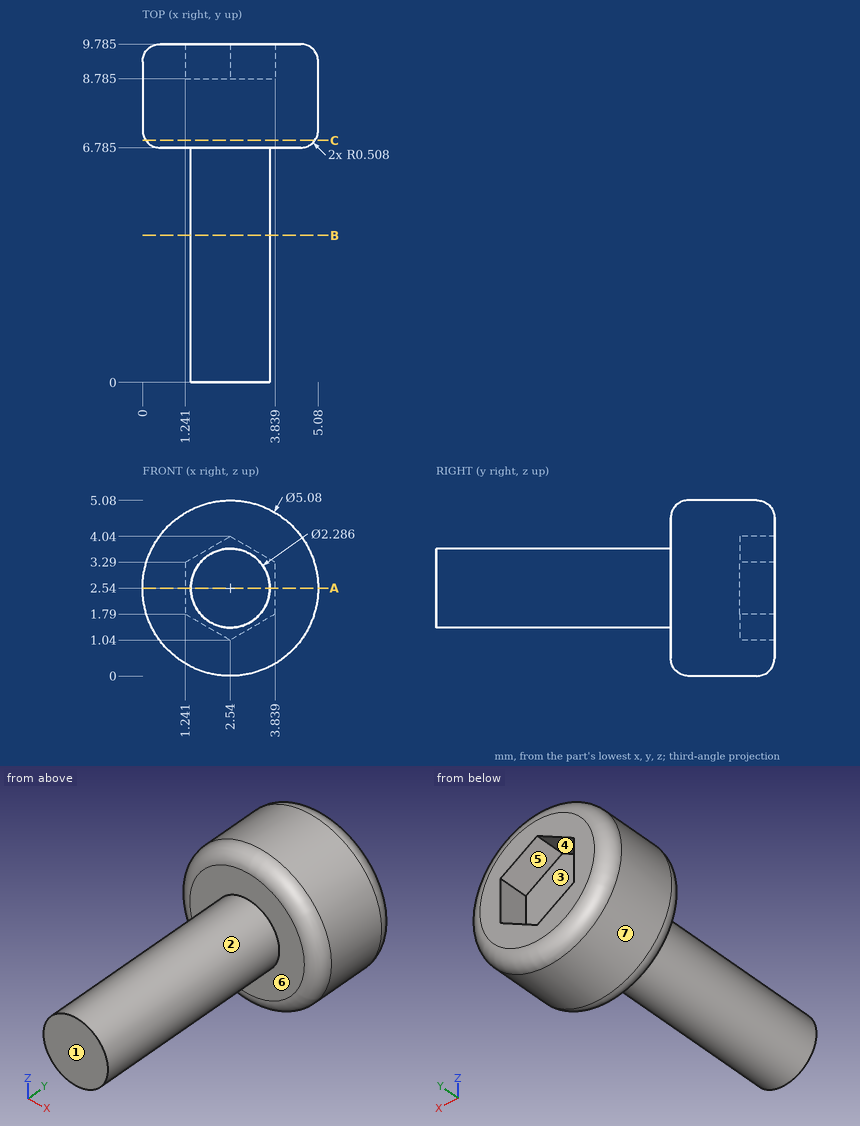
Source: three-view drawing plus pictorial views. Frame: mm from the lowest corner of the part. A direction names the side the tool comes from. Give positions to 0.01 mm unless a question says otherwise; leave off trailing zeros. Write each loop counter-clockwise with the first axis right and the second up, starting at its lowest first coordinate (ties: lowest second). Pieces come first, ordered by that corner, then holes.
(1) Cut plane C-C, the plane y = 7. Return loops of the section in (x, z), then the cut area to 3 significant figures.
(2) Cut plane A-A, the plane z = 2.54. Return loops of the section in (x, y) (3 decimals), then the cut area to 3 significant figures.
(3) First-contact query: P1, Ø3, axis at x = 4, y = 7.5, coming from the +Z side; P2, Ø3, axis at y = 1.5, z = 3.5, coming from the +X side; P3, Ø1.5, axis at y = 4, z = 0.5, coming from the +X side; P4, Ø2, axis at x = 1, y = 2.5, coming from the -Z side. Flat tips, straight axial feed; report the tip coordinate or a pass-through.
(4) Ray query, line 1 (Z direction, x = 2.5, y = 0.5); line 2 (X direction, y = 9.25, z = 2.15); line 3 (Y direction, x = 0.6, z = 2.65) (3 decimals). Return the intervals inside material, ascending.
(5) Mould query, pull axis X, two halves, no side actions, for the marked faces 4, 5, 6 and 7. Classes: released by +X, released by -X, zero draft, split by the parting line, or undercut.
(6) Access query for the marked faces 1, 2 and 3. Directions: +Z, -Z, +X, -X, +Y, -Y. A direction counts if a zero-diameter tool reaches every point of the face in a straight line with its end or side. Return the directions, or none.
(7) Cut plane B-B, the plane y = 4.25. Return loops of the section in (x, z).
Values follow:
1. outline: circle Ø4.89 at (2.54, 2.54)
1. area: 18.8 mm2
2. outline: (0, 7.293) arc R0.508 ccw to (0.508, 6.785) - (1.397, 6.785) - (1.397, 0) - (3.683, 0) - (3.683, 6.785) - (4.572, 6.785) arc R0.508 ccw to (5.08, 7.293) - (5.08, 9.277) arc R0.508 ccw to (4.572, 9.785) - (3.839, 9.785) - (3.839, 8.785) - (1.241, 8.785) - (1.241, 9.785) - (0.508, 9.785) arc R0.508 ccw to (0, 9.277) - close
2. area: 27.9 mm2
3. P1: stops at z = 5.08
3. P2: stops at x = 3.68
3. P3: passes through
3. P4: stops at z = 1.53
4. line 1: z = 1.4 to 3.68
4. line 2: x = 0.03 to 1.24, 3.84 to 5.05
4. line 3: y = 6.785 to 9.785
5. face 4: undercut
5. face 5: undercut
5. face 6: zero draft
5. face 7: split by the parting line
6. face 1: +Z, -Z, +X, -X, -Y
6. face 2: -Y
6. face 3: +Y
7. outline: circle Ø2.29 at (2.54, 2.54)
